Check sheet for the modelled part. Datum: model origin and axes. Units: mm. Face numbers are marked on the shaded views. Give positions to 0.01 mm unless a question says otherwise; leave off trailing zeros. Order: outer loops, then holes, each group sorted by start corner. A loop starts at its lowest first (then second) coordinate and runs counter-clockwise, first axis right, second up.
Item 1: Sectioned sample at D-D on z = 12.5. Record the boundary of the cut face in (x, y), and give its area (3 significant figures).
Item 2: Gauge pin test, flat ends, axial feed: P1, Ø14, axis at x = -33.2, y = 13.14, coming from the -Z side; P2, Ø3, axis at x = 37.5, z = 7.5, coming from the +Y side; P3, Ø4, axis at x = 20, z = 17, coming from the +Y side. Record the tip position at first contact, or that the pin passes through.
Item 3: Sectioned sample at A-A on y = 8.5. Record the boundary of the cut face in (x, z), and give its area (3 significant figures).
Item 4: Release check for a two-part mould opening along Y. For the marked faces 1, 2 and 3 record: released by +Y, released by -Y, zero draft, split by the parting line, or undercut.
Item 5: Sectioned sample at C-C on z = 50. Record the boundary of the cut face in (x, y).
Item 6: Sectioned sample at B-B on x = 37.5. Record the boundary of the cut face in (y, z), and give its area (3 significant figures).
Item 7: Material ranges on line 1 along Z through (x, y) = (-26, 9.5); line 2 along Y through (x, z) = (-37, 17); line 3 along Y through (x, z) = (-31, 21), recorded low to high.
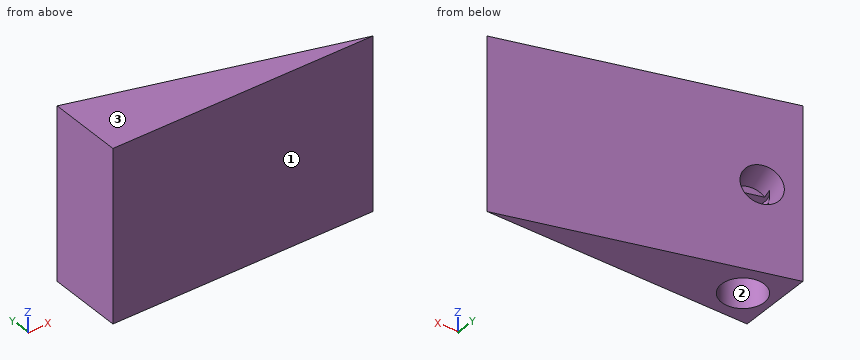
from build123d import *

# Parameters (mm, degrees)
BOSS_EXTRUDE1_DEPTH = 70
SKETCH4_R           = 7.747265665
CUT_EXTRUDE1_DEPTH  = 13
SKETCH7_R           = 8.715693707
CUT_EXTRUDE2_DEPTH  = 40


with BuildPart() as part:
    # Sketch1 → Boss-Extrude1 (new body)
    with BuildSketch(Plane.XY):
        Polygon((-44.780066958, 0), (61.341290068, 0), (-44.780066958, 30.254301436), align=None)
    extrude(amount=BOSS_EXTRUDE1_DEPTH)

    # Sketch4 → Cut-Extrude1 (cut)
    with BuildSketch(Plane(origin=(4.610887587, 16.173357987, 0), x_dir=(0.961681983, -0.274167401, 0), z_dir=(0.274167401, 0.961681983, 0))):
        with Locations((-37.136646247, -35)):
            Circle(SKETCH4_R)
    extrude(amount=-CUT_EXTRUDE1_DEPTH, mode=Mode.SUBTRACT)

    # Sketch7 → Cut-Extrude2 (cut)
    with BuildSketch(Plane(origin=(0, 0, 0), x_dir=(-1, 0, 0), z_dir=(0, 0, -1))):
        with Locations((33.204170233, 13.141177122)):
            Circle(SKETCH7_R)
    extrude(amount=-CUT_EXTRUDE2_DEPTH, mode=Mode.SUBTRACT)


solid = part.part
Report:
1. outline: (-44.78, 0) - (61.34, 0) - (-44.78, 30.25) - close; hole circle Ø17.43 at (-33.2, 13.14)
1. area: 1,370 mm2
2. P1: stops at z = 40
2. P2: stops at y = 7.22
2. P3: stops at y = 12.36
3. outline: (-44.78, 0) - (-40.58, 0) - (-40.58, 40) - (-25.83, 40) - (-25.83, 0) - (31.53, 0) - (31.53, 70) - (-44.78, 70) - close
3. area: 4,750 mm2
4. face 1: released by -Y
4. face 2: undercut
4. face 3: zero draft
5. outline: (-44.78, 0) - (61.34, 0) - (-44.78, 30.25) - close
6. outline: (0, 0) - (6.8, 0) - (6.8, 70) - (0, 70) - close
6. area: 476 mm2
7. line 1: z = 40 to 70
7. line 2: y = 0 to 5.3, 20.99 to 28.04
7. line 3: y = 0 to 4.71, 21.57 to 26.33
